Input: part model. Units: mm. Frame: model coordinates. Face numbers are marked on the shaded views. A direction names the side the tool comes from. Round coordinates to 2 decimals unless told otherwise and drop trailing zeros. Loops run counter-clockwise (first coordinate to the right, second up) from the corner with the lowest first, then second, coordinate; pieces in that order, holes last. Notation, with made-up numbers: M 29.5,47.25 L 76.5,47.25 A15 ccw 76.5,71.25 Z; hole C 83,86 d2. An arc over 180 degrees is marked long. Put each result on its own line as item: value. Start each with the question number.
1) Section C-C on x = -16. Output: boundary loops of the cut face in (y, z).
2) Section B-B on y = 7.62. Output: boundary loops of the cut face in (x, z), plus the area to 3 significant figures.
3) Reachability of the marked faces 1 and 2 from +Z, -Z, +X, -X, +Y, -Y: full face, straight path, thin tool, end or side. Return the list, or none.
4) Line query: probe 1 along Z at (x, y) = (-29.5, 4.5); probe 2 along Y at (x, z) = (-27, -38); probe 3 along Y at (x, z) = (-25.4, 0.5). Output: solid intervals per line, ascending.
5) Section D-D on z = -35. Output: boundary loops of the cut face in (x, y).
6) Pin query (flat end, axial travel): pin 1 (10 mm diameter, centred on x = -11, z = -26, fed in from +Y); pin 2 (0.5 mm diameter, centred on y = 4.5, z = -39, fed in from +X); pin 3 (0.8 mm diameter, centred on x = -7, y = 1, fed in from +Z). Return the tip coordinate at first contact, or that it passes through.
7) Section A-A on x = -25.4. Output: boundary loops of the cut face in (y, z).
Autodesk Inventor part; units mm, degrees
ref_plane "YZ Plane" through (0, 0, 0) normal (1, 0, 0) x (0, 1, 0)
ref_plane "XZ Plane" through (0, 0, 0) normal (0, 1, 0) x (-1, 0, 0)
ref_plane "XY Plane" through (0, 0, 0) normal (0, 0, 1) x (1, 0, 0)
sketch "Sketch1" plane through (0, 0, 0) normal (0, 1, 0) x (-1, 0, 0)
  line L0 (0, 0) -> (50.8, 0)
  line L1 (50.8, 0) -> (50.8, -38.354)
  line L2 (50.8, -38.354) -> (0, -38.354)
  line L3 (0, -38.354) -> (0, 0)
  dimension "d0" = 50.8
  dimension "d1" = 38.354
extrude "Extrusion1" add sketch "Sketch1" along normal blind 1.5875
sketch "Sketch2" plane through (-50.8, 0, 0) normal (0, 0, 1) x (1, 0, 0)
  line L0 (50.8, 0) -> (0, 0)
  line L1 (50.8, 0) -> (38.1, 0)
  line L2 (38.1, 0) -> (12.7, 0)
  line L3 (12.7, 0) -> (12.7, 12.7)
  line L4 (12.7, 12.7) -> (38.1, 12.7)
  line L5 (38.1, 12.7) -> (38.1, 0)
  line L6 (50.8, 1.5875) -> (0, 1.5875)
  dimension "d4" = 12.7
  dimension "d5" = 25.4
  dimension "d6" = 12.7
extrude "Extrusion2" add sketch "Sketch2" along normal blind 1.5875
sketch "Sketch3" plane through (0, 0, -38.354) normal (0, 0, -1) x (-1, 0, 0)
  line L0 (0, 0) -> (0, 1.5875)
  line L1 (12.7, 0) -> (0, 0)
  line L2 (0, 0) -> (12.7, 0)
  line L3 (12.7, 0) -> (38.1, 0)
  line L4 (38.1, 0) -> (38.1, 12.7)
  line L5 (38.1, 12.7) -> (12.7, 12.7)
  line L6 (12.7, 12.7) -> (12.7, 0)
  dimension "d9" = 12.7
  dimension "d10" = 25.4
  dimension "d11" = 12.7
  dimension "d12" = 25.4
extrude "Extrusion3" add sketch "Sketch3" along normal blind 1.5875
sketch "Sketch4" plane through (0, 0, -39.9415) normal (0, 0, -1) x (-1, 0, 0)
  circle A0 centre (25.4, 7.62) radius 2.667
  line L0 (38.1, 0) -> (38.1, 12.7)
  line L1 (38.1, 12.7) -> (12.7, 12.7)
  point P0 (0, 0)
  dimension "d15" = 12.7
  dimension "d16" = 5.08
  dimension "d17" = 5.334
extrude "Extrusion4" cut sketch "Sketch4" against normal blind 50.8
fillet "Fillet1" radius 1.27 2 edges at (-25.4, 0, -39.9415) (-25.4, 0, 1.5875)
properties part number "L1 Gearbox Cover Top"
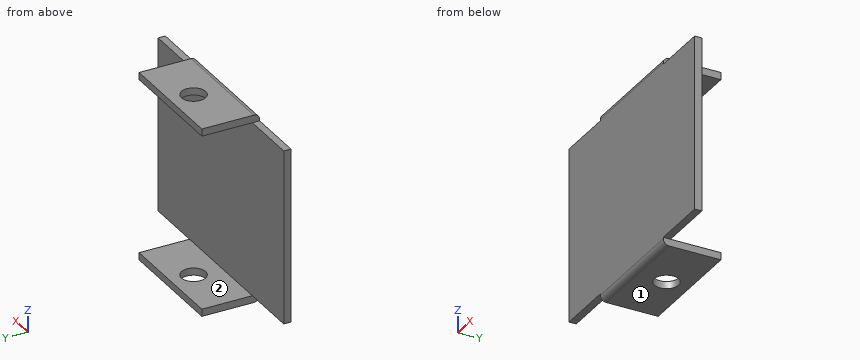
Geometry results:
1. outline: M 0,-38.67 A1.27 ccw 1.27,-39.94 L 12.7,-39.94 L 12.7,-38.35 L 1.59,-38.35 L 1.59,0 L 12.7,0 L 12.7,1.59 L 1.27,1.59 A1.27 ccw 0,0.32 Z
2. outline: M -38.1,-39.94 L -28.07,-39.94 L -28.07,-38.35 L -38.1,-38.35 Z; M -38.1,0 L -28.07,0 L -28.07,1.59 L -38.1,1.59 Z; M -22.73,-39.94 L -12.7,-39.94 L -12.7,-38.35 L -22.73,-38.35 Z; M -22.73,0 L -12.7,0 L -12.7,1.59 L -22.73,1.59 Z
2. area: 63.7 mm²
3. face 1: -Z, +X, -X, +Y, -Y
3. face 2: +X, -X, +Y
4. probe 1: z = -39.94 to -38.35, 0 to 1.59
4. probe 2: y = 0 to 1.59
4. probe 3: y = 0.01 to 4.95, 10.29 to 12.7
5. outline: M -50.8,0 L 0,0 L 0,1.59 L -50.8,1.59 Z
6. pin 1: stops at y = 1.59
6. pin 2: stops at x = -12.7
6. pin 3: stops at z = 0
7. outline: M 0,-38.67 A1.27 ccw 1.27,-39.94 L 4.95,-39.94 L 4.95,-38.35 L 1.59,-38.35 L 1.59,0 L 4.95,0 L 4.95,1.59 L 1.27,1.59 A1.27 ccw 0,0.32 Z; M 10.29,-39.94 L 12.7,-39.94 L 12.7,-38.35 L 10.29,-38.35 Z; M 10.29,0 L 12.7,0 L 12.7,1.59 L 10.29,1.59 Z
